For this review, take the finished solid that the model builds, in its own axes (mm). A direction names the side the tool comes from. Round coordinates to 2 decimals unless told otherwise and drop trailing zeros. Write each loop counter-clockwise with the first axis right and the second up, starting at its lowest first coordinate (ties: lowest second). Pieces come first, ordered by that corner, then holes. Notation, with made-up numbers: (51.5, -16.75) -> (66.5, -16.75) arc R26 ccw to (66.5, 11.25) -> close; hole circle Ø5 at (27.25, 55). An arc over 180 degrees is marked (long way). Answer as CSV lines item,"result". Start each with the question number.
Item 1: Mouldability with a two-part tool opening along Z and no side actions: class faces 4 (the cylindrical face through (-14.115, -0.028, -1.121)), 5 (the cylindrical face through (10.2, 0, 3.1)), 6 (the cylindrical face through (-294.277, -0.028, 57.352)), 7 (the cylindrical face through (-136.43, -0.03, -7.38)) as +Z half, -Z half, draft (parallel to the pull), parting line (faces both ways), or undercut.
Item 2: Wall thickness on probe 1 along Z at (x, y) = (-372, -0.75); probe 2 along X at (y, z) = (-1.6, 66); probe 3 along X at (y, z) = (-1, 71.5): over which ranges is each line inside the solid? List them lowest first. Write a range as from..to.
Item 3: For pin 1 Ø1 at (x, y) = (-317.5, -1) entering from -Z, flat-tipped, find the tip position at first contact; note if it passes through.
Item 4: Take a section at C-C on z = 78. Give the boundary of the cut face in (x, y), then the cut area to 3 significant figures.
Item 5: Take a section at A-A on x = -244. Give the boundary of the cut face in (y, z), then the cut area to 3 significant figures.
Item 6: Machinability: for faces 1 (the flat face through (-388.86, -0.03, 97.46)), 2 (the cylindrical face through (-356.923, -0.028, 62.276)), 3 (the flat face through (-266.766, -0.028, 28.672)), which of the approach directions +Z, -Z, +X, -X, +Y, -Y give a long, thin tool a straight path to every point of the face, cutting with its end or side? Answer none if there is none.
Item 7: Take a section at B-B on y = 0.5. Count the separate pieces of the cut face and the enclosed holes in it, then the cut area to 3 significant figures.
Autodesk Inventor part; units mm, degrees
ref_plane "YZ Plane" through (0, 0, 0) normal (1, 0, 0) x (0, 1, 0)
ref_plane "XZ Plane" through (0, 0, 0) normal (0, 1, 0) x (-1, 0, 0)
ref_plane "XY Plane" through (0, 0, 0) normal (0, 0, 1) x (1, 0, 0)
sketch "スケッチ1" plane through (0, 0, 0) normal (0, 1, 0) x (-1, 0, 0)
  arc A0 (395.0712, 101.8969) -> (435.2675, 137.2475) centre (306.3013, 243.3635) ccw
  arc A1 (365.0957, 97.3477) -> (365.7216, 93.5054) centre (366.6087, 95.622) ccw
  arc A2 (369.5386, 100.605) -> (365.0957, 97.3477) centre (385.9519, 73.5593) ccw
  arc A3 (385.8674, 109.4763) -> (369.5386, 100.605) centre (470.4646, -65.7001) ccw
  arc A4 (385.8674, 109.4763) -> (396.1841, 114.479) centre (-1159.575, 3309.6389) ccw
  arc A5 (396.1841, 114.479) -> (414.939, 124.7316) centre (296.9263, 318.331) ccw
  arc A6 (414.939, 124.7316) -> (434.3408, 138.1953) centre (311.0977, 295.0828) ccw
  arc A7 (435.2675, 137.2475) -> (434.3408, 138.1953) centre (434.7527, 137.6711) ccw
  arc A8 (319.6761, 45.1314) -> (390.0033, 84.5371) centre (233.4832, 281.4189) ccw
  arc A9 (273.0796, 42.1444) -> (277.153, 40.2312) centre (280.7432, 53.1684) ccw
  arc A10 (273.4497, 49.6709) -> (273.0796, 42.1444) centre (275.6154, 45.792) ccw
  arc A11 (281.147, 53.127) -> (273.4497, 49.6709) centre (297.0704, 7.3635) ccw
  arc A12 (307.9726, 61.0464) -> (281.147, 53.127) centre (377.3682, -223.4121) ccw
  arc A13 (307.9726, 61.0464) -> (324.6713, 65.1488) centre (-955.196, 5238.8807) ccw
  circle A14 centre (20.1088, -0.8575) radius 6
  circle A15 centre (130.7072, -5.574) radius 6
  arc A16 (390.0033, 84.5371) -> (388.4453, 88.078) centre (388.7587, 86.1027) ccw
  line L0 (388.4453, 88.078) -> (384.6663, 87.4784)
  arc A17 (382.4737, 92.8975) -> (384.6663, 87.4784) centre (384.1962, 90.4413) ccw
  arc A18 (281.147, 53.127) -> (273.4497, 49.6709) centre (297.0704, 7.3635) ccw
  line L1 (277.153, 40.2312) -> (280.996, 39.1647)
  arc A19 (281.136, 33.4257) -> (280.996, 39.1647) centre (280.1938, 36.274) ccw
  line L2 (281.136, 33.4257) -> (251.9878, 23.784)
  arc A20 (232.2409, 19.4065) -> (251.9878, 23.784) centre (220.5829, 118.7246) ccw
  arc A21 (202.438, 16.5387) -> (232.2409, 19.4065) centre (148.7903, 730.3461) ccw
  arc A22 (125.7464, 14.4013) -> (202.438, 16.5387) centre (141.4444, 828.0876) ccw
  arc A23 (84.4867, 15.2639) -> (125.7464, 14.4013) centre (372.4747, 12803.2702) ccw
  arc A24 (84.4867, 15.2639) -> (17.3799, 13.5681) centre (68.6653, -687.2803) ccw
  arc A25 (17.3799, 13.5681) -> (-2.611, 10.3374) centre (25.867, -102.4131) ccw
  arc A26 (-2.611, 10.3374) -> (-8.1443, -6.881) centre (0, 0) ccw
  arc A27 (-8.1443, -6.881) -> (0.1105, -13.8465) centre (16.4695, 13.9147) ccw
  arc A28 (0.1105, -13.8465) -> (28.2747, -25.3165) centre (53.2618, 76.3513) ccw
  arc A29 (28.2747, -25.3165) -> (76.0298, -30.4027) centre (70.8911, 148.0818) ccw
  arc A30 (76.0298, -30.4027) -> (101.7324, -28.9004) centre (63.5115, 404.3974) ccw
  arc A31 (101.7324, -28.9004) -> (312.4116, 29.4193) centre (48.6916, 572.4065) ccw
  arc A32 (312.4116, 29.4193) -> (311.5978, 33.2175) centre (311.5379, 31.2183) ccw
  line L3 (311.5978, 33.2175) -> (304.4845, 33.4306)
  arc A33 (303.5463, 39.2476) -> (304.4845, 33.4306) centre (304.5744, 36.4292) ccw
  line L4 (303.5463, 39.2476) -> (319.6761, 45.1314)
  line L5 (365.7216, 93.5054) -> (369.4507, 91.9425)
  arc A34 (369.4958, 84.5835) -> (369.4507, 91.9425) centre (367.9046, 88.2534) ccw
  line L6 (369.4958, 84.5835) -> (324.6713, 65.1488)
  line L7 (395.0712, 101.8969) -> (382.4737, 92.8975)
  point P0 (0, 0)
  dimension "d1" = 4
extrude "押し出し2" add sketch "スケッチ1" along normal mid plane 4
sketch "スケッチ2" plane through (0, -2, 0) normal (0, -1, 0) x (1, 0, 0)
  circle A0 centre (-372.2064, 97.2423) radius 3.25
  circle A1 centre (-405.9401, 114.7361) radius 3.25
  line L0 (-405.9401, 114.7361) -> (-372.2064, 97.2423)
  point P0 (0, 0)
  dimension "d6" = 6.5
  dimension "d7" = 6.5
  dimension "d8" = 38
extrude "押し出し3" cut sketch "スケッチ2" against normal blind 10
sketch "スケッチ3" plane through (0, -2, 0) normal (0, -1, 0) x (1, 0, 0)
  circle A0 centre (-357.6123, 68.7377) radius 3
  circle A1 centre (-285.7217, 47.1567) radius 3
  point P0 (0, 0)
extrude "押し出し4" cut sketch "スケッチ3" against normal through all
properties part number "newbracket2"
Output values:
1,face 4,"undercut"
1,face 5,"parting line"
1,face 6,"+Z half"
1,face 7,"undercut"
2,probe 1,"z = 71.48..94, 100.49..102.07"
2,probe 2,"x = -363.31..-358.84, -356.39..-326.63"
2,probe 3,"x = -372.03..-358.78, -356.44..-339.32"
3,pin 1,"stops at z = 44.16"
4,outline,"(-381.41, -2) -> (-354.31, -2) -> (-354.31, 2) -> (-381.41, 2) -> close"
4,area,"108 mm^2"
5,outline,"(-2, 1.23) -> (2, 1.23) -> (2, 21.51) -> (-2, 21.51) -> close"
5,area,"81.1 mm^2"
6,face 1,"-X, +Y, -Y"
6,face 2,"-Z, -X, +Y, -Y"
6,face 3,"+X, +Y, -Y"
7,separate pieces,"1"
7,enclosed holes,"6"
7,area,"12,500 mm^2"
